Verification items for this drawing (mm, ordinates from the low corner). Round coordinates to 2 decimals unless told otherwise and drop trailing zeros. Write each loop counter-clockwise with the first axis right and the second up, starting at its lowest first coordinate (ties: lowest second). Pieces come first, ordered by that corner, then holes. Notation, with made-up numbers: (39.5, -40) -> (92.5, -40) arc R11 cw to (92.5, -20) -> close; hole circle Ø6 at (-34.75, 66.25). An arc over 180 degrees is marked (long way). Return JSON: item names as keys, results as strings. Group by question number.
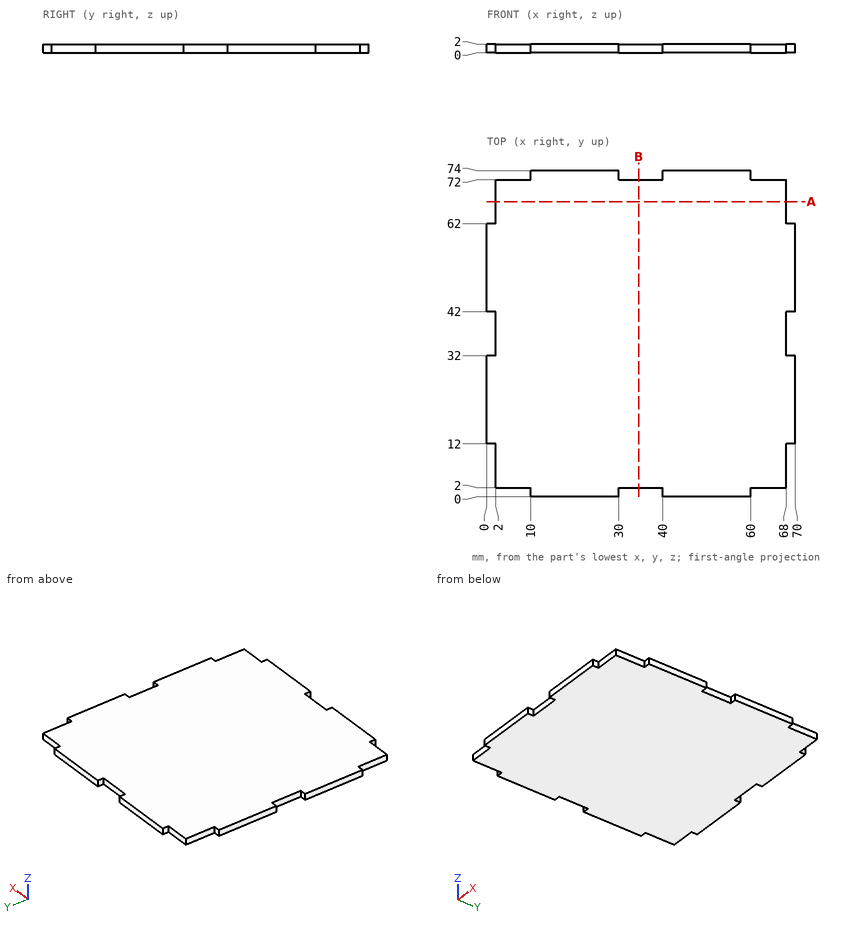
1) Sectioned sample at A-A on y = 67. Enter the section's corners in (x, z), and give its area (3 significant figures).
2) Sectioned sample at B-B on x = 34.5. Enter the section's corners in (y, z).
3) Material ranges on probe 1 along Y at (x, z) = (67.5, 1.4); probe 2 along X at (y, z) = (67.5, 1.7), recorded low to high. Write a range as [from, to].
4) Go/stop test with flat-tipped pins: P1, Ø0.6, axis at x = 1, z = 1, coming from the +Y side; P2, Ø0.6, axis at y = 39, z = 1, coming from the +X side; P3, Ø1, axis at y = 73, z = 1, coming from the -X side. Record where each tip stops, or that it passes through.
Evaluation:
{
 "1": {"outline": "(2, 0) -> (68, 0) -> (68, 2) -> (2, 2) -> close", "area": "132 mm2"},
 "2": {"outline": "(2, 0) -> (72, 0) -> (72, 2) -> (2, 2) -> close"},
 "3": {"probe 1": "y = [2, 72]", "probe 2": "x = [2, 68]"},
 "4": {"P1": "stops at y = 62", "P2": "stops at x = 68", "P3": "stops at x = 10"}
}
